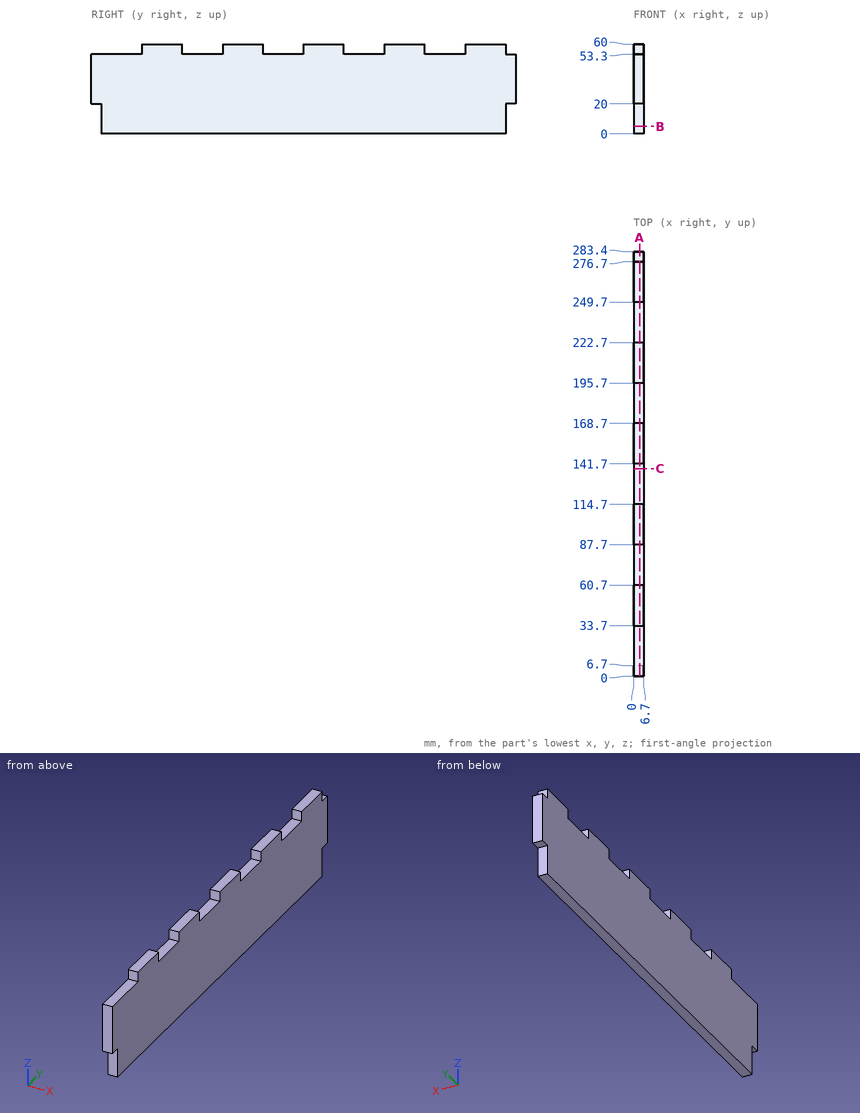
For this review, use the dimensioned drawing (mm, ordinates from the lowest corner) and the shaded views. Round coordinates to 2 decimals unless told otherwise and drop trailing zeros. Order: outer loops, then holes, each group sorted by start corner. A loop starts at its lowest first (then second) coordinate and runs counter-clockwise, first axis right, second up. Notation, with made-up numbers: (62, -38) -> (113, -38) arc R19 ccw to (113, -5) -> close; hole circle Ø6 at (78.25, 67). An arc over 180 degrees is marked (long way). Write item = value, one per line. Start each with the question number.
Item 1: Clearance check with flat-ended pins moving along their axes: pin 1 Ø1.5 at (x, z) = (3, 52) entering from -Y; pin 2 Ø3.5 at (x, y) = (4.5, 235) entering from +Z; pin 3 Ø3.5 at (x, z) = (3, 57) entering from +Y. State where each tip first meets the part, or that it passes through.
Item 2: For line 1 along Y through (x, z) = (5.75, 55); line 2 along Z through (x, y) = (4.25, 140); line 3 along Y through (x, z) = (0.5, 13), list the stretches that pass through material, from the lowest coordinate up.
Item 3: Consider section A-A on x = 4. Write out the cut boundary in (y, z), plus the area to 3 significant figures.
Item 4: Consider section B-B on z = 5. Write out the cut boundary in (x, y).
Item 5: Consider section C-C on y = 138.5. Write out the cut boundary in (x, z).
Conclusion:
q1.pin_1 = 0
q1.pin_2 = 53.3
q1.pin_3 = 276.7
q2.line_1 = 33.7 to 60.7, 87.7 to 114.7, 141.7 to 168.7, 195.7 to 222.7, 249.7 to 276.7
q2.line_2 = 0 to 53.3
q2.line_3 = 6.7 to 276.7
q3.outline = (0, 20) -> (6.7, 20) -> (6.7, 0) -> (276.7, 0) -> (276.7, 20) -> (283.4, 20) -> (283.4, 53.3) -> (276.7, 53.3) -> (276.7, 60) -> (249.7, 60) -> (249.7, 53.3) -> (222.7, 53.3) -> (222.7, 60) -> (195.7, 60) -> (195.7, 53.3) -> (168.7, 53.3) -> (168.7, 60) -> (141.7, 60) -> (141.7, 53.3) -> (114.7, 53.3) -> (114.7, 60) -> (87.7, 60) -> (87.7, 53.3) -> (60.7, 53.3) -> (60.7, 60) -> (33.7, 60) -> (33.7, 53.3) -> (0, 53.3) -> close
q3.area = 15,700 mm2
q4.outline = (0, 6.7) -> (6.7, 6.7) -> (6.7, 276.7) -> (0, 276.7) -> close
q5.outline = (0, 0) -> (6.7, 0) -> (6.7, 53.3) -> (0, 53.3) -> close
